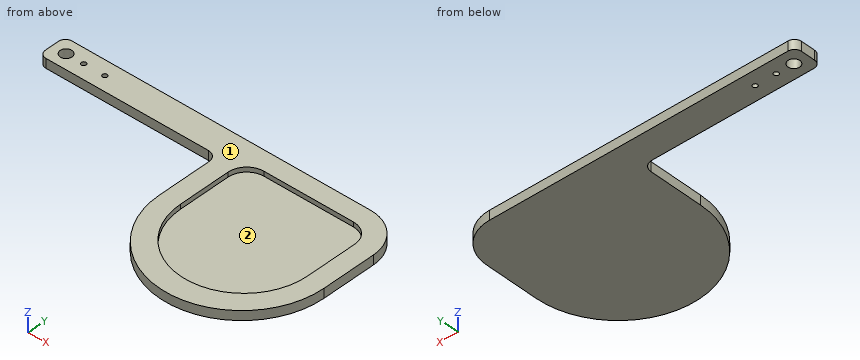
from build123d import *

# Parameters (mm, degrees)
SKETCH_1_R          = 2.5
SKETCH_1_R_2        = 1
EXTRUDE_1_DEPTH     = 4
CUT_EXTRUDE_1_DEPTH = 2


with BuildPart() as part:
    # Эскиз1 → Бобышка-Вытянуть1 (new body)
    with BuildSketch(Plane.XY):
        with BuildLine():
            Line((3, 0), (72, 0))
            ThreePointArc((72, 0), (74.828427125, -1.171572875), (76, -4))
            Line((76, -4), (76, -27))
            ThreePointArc((76, -27), (111, -62), (146, -27))
            Line((146, -27), (146, -4))
            ThreePointArc((146, -4), (141.313708499, 7.313708499), (130, 12))
            Line((130, 12), (3, 12))
            ThreePointArc((3, 12), (0.878679656, 11.121320344), (0, 9))
            Line((0, 9), (0, 3))
            ThreePointArc((0, 3), (0.878679656, 0.878679656), (3, 0))
        make_face()
        with Locations((6, 6)):
            Circle(SKETCH_1_R, mode=Mode.SUBTRACT)
        with Locations((13.5, 6)):
            Circle(SKETCH_1_R_2, mode=Mode.SUBTRACT)
        with Locations((22.5, 6)):
            Circle(SKETCH_1_R_2, mode=Mode.SUBTRACT)
    extrude(amount=EXTRUDE_1_DEPTH)

    # Эскиз2 → Вырез-Вытянуть1 (cut)
    with BuildSketch(Plane.XY.offset(4)):
        with BuildLine():
            Line((92, 4), (130, 4))
            ThreePointArc((130, 4), (135.656854249, 1.656854249), (138, -4))
            Line((138, -4), (138, -26))
            ThreePointArc((138, -26), (111, -53), (84, -26))
            Line((84, -26), (84, -4))
            ThreePointArc((84, -4), (86.343145751, 1.656854249), (92, 4))
        make_face()
    extrude(amount=-CUT_EXTRUDE_1_DEPTH, mode=Mode.SUBTRACT)


solid = part.part
CAD build for the part. Positions are in the model's coordinates, mm. Face numbers are marked on the shaded views. Coordinates: 2 decimals unless noted, no trailing zeros. Order: outer loops, then holes, each group sorted by start corner. A loop starts at its lowest first (then second) coordinate and runs counter-clockwise, first axis right, second up. Notation, with made-up numbers: (86, 48.25) -> (145, 48.25) arc R17 ccw to (145, 53.25) -> close; hole circle Ø10 at (66, -15.75). An arc over 180 degrees is marked (long way). Answer in a Markdown table with one row per item.
1) Mould opens along X. For the marked faces 1 and 2 say: pulls with the +X half, pulls with the -X half, needs draft (parallel to the pull), parting line crosses it, or undercut.
Check values:
| item | result |
|---|---|
| face 1 | needs draft |
| face 2 | undercut |
2) Band-saw the part on D-D (x = 118). List the corners of the cut face in (y, z).
Check values:
| item | result |
|---|---|
| outline | (-61.29, 0) -> (12, 0) -> (12, 4) -> (4, 4) -> (4, 2) -> (-52.08, 2) -> (-52.08, 4) -> (-61.29, 4) -> close |
3) Flat gauge pins, fed straight in: P1, Ø4.5, axis at x = 6, y = 6, coming from the -Z side; P2, Ø1.6, axis at y = -13, z = 3, coming from the -X side; P3, Ø0.6, axis at x = 120, z = 3, coming from the -Y side; P4, Ø2, axis at x = 54, z = 2, coming from the -Y side. Where does each tip first touch, or does it go through?
Check values:
| item | result |
|---|---|
| P1 | through |
| P2 | x = 76 |
| P3 | y = -60.9 |
| P4 | y = 0 |
4) Band-saw the part on B-B (z = 0.65). List the corners of the cut face in (x, y).
Check values:
| item | result |
|---|---|
| outline | (0, 3) arc R3 ccw to (3, 0) -> (72, 0) arc R4 cw to (76, -4) -> (76, -27) arc R35 ccw to (146, -27) -> (146, -4) arc R16 ccw to (130, 12) -> (3, 12) arc R3 ccw to (0, 9) -> close; hole circle Ø5 at (6, 6); hole circle Ø2 at (13.5, 6); hole circle Ø2 at (22.5, 6) |
5) Band-saw the part on A-A (x = 6). List the corners of the cut face in (y, z).
Check values:
| item | result |
|---|---|
| outline | (0, 0) -> (3.5, 0) -> (3.5, 4) -> (0, 4) -> close; (8.5, 0) -> (12, 0) -> (12, 4) -> (8.5, 4) -> close |
6) Band-saw the part on C-C (y = -23). List the corners of the cut face in (x, z).
Check values:
| item | result |
|---|---|
| outline | (76, 0) -> (146, 0) -> (146, 4) -> (138, 4) -> (138, 2) -> (84, 2) -> (84, 4) -> (76, 4) -> close |
7) Drill centre lines: line 1 (Y direction, x = 22.5, z = 2.9); line 2 (Y direction, x = 110.5, z = 2.45); line 3 (X direction, y = -7.5, z = 2.75). Where is each one in solid material? Low to high.
Check values:
| item | result |
|---|---|
| line 1 | 0 to 5, 7 to 12 |
| line 2 | -62 to -53, 4 to 12 |
| line 3 | 76 to 84, 138 to 146 |
